```python
from build123d import *

# Parameters (mm, degrees)
EXTRUDE_1_DEPTH = 20
FILLET_2_R      = 10
FILLET_1_R      = 5


with BuildPart() as part:
    # 草圖1 → 填料-伸長1 (new body)
    with BuildSketch(Plane.XY):
        Polygon((0, 0), (0, 15), (10, 15), (10, 20), (15, 20), (15, 10), (35, 10), (35, 5), (20, 5), (20, -5), (5, -5), (5, 0), align=None)
    extrude(amount=EXTRUDE_1_DEPTH)

    # 圓角2
    fillet_2_edges = [part.edges().sort_by_distance(p)[0] for p in [
        (35, 7.5, 0),
        (35, 7.5, 20),
    ]]
    fillet(fillet_2_edges, radius=FILLET_2_R - 0.0001)  # a hair under: the kernel refuses the full size

    # 圓角1
    fillet_1_edges = [part.edges().sort_by_distance(p)[0] for p in [
        (20, 5, 10),
        (15, 10, 10),
    ]]
    fillet(fillet_1_edges, radius=FILLET_1_R)


solid = part.part
```
The model under review builds one solid part; all positions refer to its coordinate system, in mm. A direction names the side the tool comes from. Round coordinates to 2 decimals unless told otherwise and drop trailing zeros. Loops run counter-clockwise (first coordinate to the right, second up) from the corner with the lowest first, then second, coordinate; pieces in that order, holes last. Notation, with made-up numbers: (89, -37.5) - (94, -37.5) arc R15 cw to (94, -23.5) - close; hole circle Ø9 at (43, 69). An arc over 180 degrees is marked (long way). Use a Markdown table: item, result. Add a question column.
Q1. Add section A-A (z = 16.75). State the section outline as (x, y) points.
Q2. Insertion check: pin 1 Ø5.5 at (x, z) = (2, 14) entering from -Y; pin 2 Ø12 at (y, z) = (14.5, 2.5) entering from +X; pin 3 Ø3 at (y, z) = (5, 4) entering from +X. Each pin has a flat end and moves straight along its axis. Give the tip position at first contact, or say it passes through.
Q3. For probe 1 along X at (y, z) = (-1.25, 3); probe 2 along Y at (x, z) = (31, 11); probe 3 along Y at (x, z) = (4.5, 6.5), list the stretches that pass through material, from the lowest coordinate up.
Q4. Machinability: for faces 1 (the face through (5, 15, 10)), 2 (the face through (29, 5, 10)), 3 (the face through (5, -3, 10)), which of the approach directions +Z, -Z, +X, -X, +Y, -Y give a long, thin tool a straight path to every point of the face, cutting with its end or side? Answer none if there is none.
Q5. Add section D-D (z = 8.25). State the section outline as (x, y) points.
Q6. Add section B-B (x = 22). State the section outline as (y, z) points, plus the area to 3 significant figures.
Worked answers:
| question | item | result |
|---|---|---|
| 1 | outline | (0, 0) - (5, 0) - (5, -5) - (20, -5) - (20, 0) arc R5 cw to (25, 5) - (32.38, 5) - (32.38, 10) - (20, 10) arc R5 cw to (15, 15) - (15, 20) - (10, 20) - (10, 15) - (0, 15) - close |
| 2 | pin 1 | y = 0 |
| 2 | pin 2 | x = 34.36 |
| 2 | pin 3 | x = 33.93 |
| 3 | probe 1 | 5 to 20 |
| 3 | probe 2 | 5 to 10 |
| 3 | probe 3 | 0 to 15 |
| 4 | face 1 | +Z, -Z, -X, +Y |
| 4 | face 2 | +Z, -Z, +X, -Y |
| 4 | face 3 | +Z, -Z, -X, -Y |
| 5 | outline | (0, 0) - (5, 0) - (5, -5) - (20, -5) - (20, 0) arc R5 cw to (25, 5) - (34.85, 5) - (34.85, 10) - (20, 10) arc R5 cw to (15, 15) - (15, 20) - (10, 20) - (10, 15) - (0, 15) - close |
| 6 | outline | (4, 0) - (10, 0) - (10, 20) - (4, 20) - close |
| 6 | area | 120 mm² |
